```python
from build123d import *

# Parameters (mm, degrees)
BOSS_EXTRUDE1_DEPTH = 50
SKETCH3_R           = 25
BOSS_EXTRUDE2_DEPTH = 17.5
HOLE1_D             = 25
HOLE2_D             = 10
CUT_EXTRUDE1_DEPTH  = 91.34873625


with BuildPart() as part:
    # Sketch1 → Boss-Extrude1 (new body)
    with BuildSketch(Plane.XY):
        Polygon((0, 9), (0, -9), (-20.176914536, -9), (-59.301270189, -31.588457268), (-68.301270189, -16), (-25, 9), align=None)
    extrude(amount=BOSS_EXTRUDE1_DEPTH)

    # Sketch3 → Boss-Extrude2 (add, symmetric)
    with BuildSketch(Plane(origin=(0, 0, 0), x_dir=(1, 0, 0), z_dir=(0, 1, 0))):
        with Locations(Location((0, -25, 0), (0, 0, 270))):
            Circle(SKETCH3_R)
    extrude(amount=BOSS_EXTRUDE2_DEPTH, both=True)

    # Hole1 (through all)
    with Locations(Plane(origin=(0, 17.5, 0), x_dir=(1, 0, 0), z_dir=(0, 1, 0))):
        with Locations((0, -25)):
            Hole(HOLE1_D / 2)

    # Hole2 (through all)
    with Locations(Plane(origin=(-10.147114317, 17.575317547, 0), x_dir=(0.8660254037844378, 0.5000000000000017, 0), z_dir=(-0.5000000000000016, 0.8660254037844377, 0))):
        with Locations((-57.150635095, -25)):
            Hole(HOLE2_D / 2)

    # Sketch9 → Cut-Extrude1 (cut, through all)
    with BuildSketch(Plane.XY.offset(50)):
        Polygon((-50.980762114, -6), (-42.320508076, -1), (-39.820508076, -5.330127019), (-48.480762114, -10.330127019), align=None)
    extrude(amount=-CUT_EXTRUDE1_DEPTH, mode=Mode.SUBTRACT)


solid = part.part
```
Geometry: final body of the model. Coordinates: model frame, mm. A direction names the side the tool comes from. Round coordinates to 2 decimals unless told otherwise and drop trailing zeros. Order: outer loops, then holes, each group sorted by start corner. A loop starts at its lowest first (then second) coordinate and runs counter-clockwise, first axis right, second up. Notation, with made-up numbers: (33.5, 14.25) -> (39.5, 14.25) arc R18 ccw to (39.5, 31.25) -> close; hole circle Ø7 at (16.25, -6). An arc over 180 degrees is marked (long way). Use one line per item in the form item = value.
(1) First-contact query: pin 1 Ø8 at (x, z) = (-8.5, 46) entering from -Y; pin 2 Ø3 at (y, z) = (-5, 7) entering from +X; pin 3 Ø10 at (x, z) = (-58, 30.5) entering from +Y. Flat tips, straight axial feed; report the tip coordinate or a pass-through.
Results list:
pin_1 = -17.5
pin_2 = 18.78
pin_3 = -7.17
(2) Section A-A on x = -6. Return loops of the section in (y, z).
Results list:
outline = (-17.5, 0.73) -> (-9, 0.73) -> (-9, 0) -> (9, 0) -> (9, 0.73) -> (17.5, 0.73) -> (17.5, 14.03) -> (-17.5, 14.03) -> close; (-17.5, 35.97) -> (17.5, 35.97) -> (17.5, 49.27) -> (9, 49.27) -> (9, 50) -> (-9, 50) -> (-9, 49.27) -> (-17.5, 49.27) -> close
(3) Draft query along X for faces 5 (the face through (-44.1, -7.8, 25.4)), 6 (the face through (-59.76, -11.07, 19.09)), 7 (the face through (11.5, -17.5, 19.1)). Return one class per face: pulls with the +X half, pulls with the -X half, needs draft (parallel to the pull), parting line crosses it, or undercut.
Results list:
face_5 = undercut
face_6 = pulls with the -X half
face_7 = needs draft
(4) Section C-C on y = 13.5. Return loops of the section in (x, z).
Results list:
outline = circle Ø50 at (0, 25); hole circle Ø25 at (0, 25)
(5) Ray query, probe 1 along Z at (x, y) = (0, -4.5); probe 2 along X at (y, z) = (-9, 30.5); probe 3 along X at (y, z) = (15.5, 32). Return the intervals inside material, ascending. Write a range as [from, to].
Results list:
probe_1 = [0, 12.5], [37.5, 50]
probe_2 = [-56.18, -49.25], [-46.18, -11.22], [11.22, 24.39]
probe_3 = [-24, -10.36], [10.36, 24]
(6) Section B-B on z = 18. Return loops of the section in (x, y).
Results list:
outline = (-68.3, -16) -> (-59.3, -31.59) -> (-24, -11.21) -> (-24, -17.5) -> (-10.36, -17.5) -> (-10.36, 17.5) -> (-24, 17.5) -> (-24, 9) -> (-25, 9) -> (-42.32, -1) -> (-39.82, -5.33) -> (-48.48, -10.33) -> (-50.98, -6) -> close; (10.36, -17.5) -> (24, -17.5) -> (24, 17.5) -> (10.36, 17.5) -> close
(7) Access query for faces 1 (the face through (-20, 9, 6)), 2 (the face through (-20, 9, 44)), 3 (the face through (-41.09, -3.13, 25.35)), 4 (the face through (-49.71, -8.2, 25.35)). Directions: +Z, -Z, +X, -X, +Y, -Y. A direction counts if a zero-diameter tool reaches every point of the face in a straight line with its end or side. Return the directions, or none.
Results list:
face_1 = -Z, -X, +Y
face_2 = +Z, -X, +Y
face_3 = +Z, -Z, -X
face_4 = +Z, -Z, +Y
(8) Section D-D on z = 29. Return loops of the section in (x, y).
Results list:
outline = (-68.3, -16) -> (-59.3, -31.59) -> (-53.24, -28.09) -> (-62.24, -12.5) -> close; (-57.04, -9.5) -> (-48.04, -25.09) -> (-24.68, -11.6) -> (-24.68, -17.5) -> (-11.84, -17.5) -> (-11.84, 17.5) -> (-24.68, 17.5) -> (-24.68, 9) -> (-25, 9) -> (-42.32, -1) -> (-39.82, -5.33) -> (-48.48, -10.33) -> (-50.98, -6) -> close; (11.84, -17.5) -> (24.68, -17.5) -> (24.68, 17.5) -> (11.84, 17.5) -> close
